from build123d import *

# Parameters (mm, degrees)
SKETCH1_W           = 35
SKETCH1_H           = 46
BOSS_EXTRUDE1_DEPTH = 13
SKETCH2_R           = 1.65
CUT_EXTRUDE1_DEPTH  = 26
SKETCH5_R           = 10.2
CUT_EXTRUDE2_DEPTH  = 46
SKETCH8_R           = 1.65
CUT_EXTRUDE3_DEPTH  = 26
SKETCH9_R           = 1.65
CUT_EXTRUDE4_DEPTH  = 35


with BuildPart() as part:
    # Sketch1 → Boss-Extrude1 (new body, symmetric)
    with BuildSketch(Plane(origin=(0, 0, 0), x_dir=(1, 0, 0), z_dir=(0, 1, 0))):
        Rectangle(SKETCH1_W, SKETCH1_H)
    extrude(amount=BOSS_EXTRUDE1_DEPTH, both=True)

    # Sketch2 → Cut-Extrude1 (cut)
    with BuildSketch(Plane(origin=(0, 13, 0), x_dir=(1, 0, 0), z_dir=(0, 1, 0))):
        with Locations((-13.5, 3)):
            Circle(SKETCH2_R)
        with Locations((-13.5, -19)):
            Circle(SKETCH2_R)
        with Locations((13.5, -19)):
            Circle(SKETCH2_R)
        with Locations((13.5, 3)):
            Circle(SKETCH2_R)
    extrude(amount=-CUT_EXTRUDE1_DEPTH, mode=Mode.SUBTRACT)

    # Sketch5 → Cut-Extrude2 (cut)
    with BuildSketch(Plane.XY.offset(23)):
        Circle(SKETCH5_R)
    extrude(amount=-CUT_EXTRUDE2_DEPTH, mode=Mode.SUBTRACT)

    # Sketch8 → Cut-Extrude3 (cut)
    with BuildSketch(Plane(origin=(0, 13, 0), x_dir=(1, 0, 0), z_dir=(0, 1, 0))):
        with Locations((0, 15)):
            Circle(SKETCH8_R)
    extrude(amount=-CUT_EXTRUDE3_DEPTH, mode=Mode.SUBTRACT)

    # Sketch9 → Cut-Extrude4 (cut)
    with BuildSketch(Plane.ZY.offset(17.5)):
        with Locations((7, 0)):
            Circle(SKETCH9_R)
    extrude(amount=-CUT_EXTRUDE4_DEPTH, mode=Mode.SUBTRACT)


solid = part.part
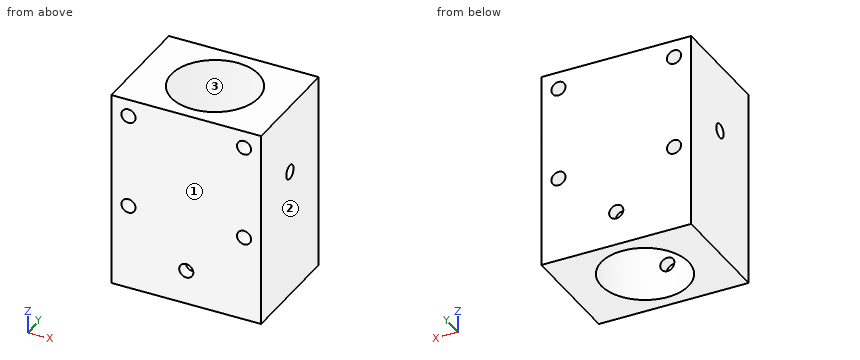
Work out the finished part from the listing and answer in its coordinate system (mm). Face numbers are marked on the shaded views. Round coordinates to 2 decimals unless told otherwise and drop trailing zeros. Loops run counter-clockwise (first coordinate to the right, second up) from the corner with the lowest first, then second, coordinate; pieces in that order, holes last. Notation, with made-up numbers: (71, 76) - (117, 76) arc R13 ccw to (117, 99) - close; hole circle Ø3 at (13, -0.75). An arc over 180 degrees is marked (long way). Use one line per item in the form item = value. Start each with the question number.
(1) Find section D-D on x = 0. Determine the outline of the cut face in (y, z), and give its area (3 significant figures).
(2) Find section B-B on x = -13.5. Determine the outline of the cut face in (y, z).
(3) Consider line 1 (Y direction, x = 0, z = -11); line 2 (Z direction, x = -13.5, y = -5); line 3 (Y direction, x = -1.5, z = 10). Determine where each line is inside the solid, lowest interval first.
(4) Determine the mould class of the marked faces 1, 2 and 3 for opening direction X: +X half, -X half, draft (parallel to the pull), parting line (faces both ways), or undercut.
(5) A flat-ended cylindrical pin translates along its axis: P1, Ø3, axis at y = 0, z = 7, coming from the +X side. Find the tip coordinate at first contact, or state that the pin passes through.
(6) Find section A-A on y = 0. Determine the outline of the cut face in (x, z).
(7) Find section C-C on z = 19. Determine the outline of the cut face in (x, y).
Answer list:
q1.outline = (-13, -23) - (-10.2, -23) - (-10.2, -16.65) - (-13, -16.65) - close; (-13, -13.35) - (-10.2, -13.35) - (-10.2, 23) - (-13, 23) - close; (10.2, -23) - (13, -23) - (13, -16.65) - (10.2, -16.65) - close; (10.2, -13.35) - (13, -13.35) - (13, 23) - (10.2, 23) - close
q1.area = 239 mm^2
q2.outline = (-13, -23) - (13, -23) - (13, -4.65) - (-13, -4.65) - close; (-13, -1.35) - (13, -1.35) - (13, 17.35) - (-13, 17.35) - close; (-13, 20.65) - (13, 20.65) - (13, 23) - (-13, 23) - close; hole circle Ø3.3 at (0, 7)
q3.line_1 = -13 to -10.2, 10.2 to 13
q3.line_2 = -23 to -4.65, -1.35 to 17.35, 20.65 to 23
q3.line_3 = -13 to -10.09, 10.09 to 13
q4.face_1 = draft
q4.face_2 = +X half
q4.face_3 = undercut
q5.P1 = through
q6.outline = (-17.5, -23) - (-10.2, -23) - (-10.2, 5.35) - (-17.5, 5.35) - close; (-17.5, 8.65) - (-10.2, 8.65) - (-10.2, 23) - (-17.5, 23) - close; (10.2, -23) - (17.5, -23) - (17.5, 5.35) - (10.2, 5.35) - close; (10.2, 8.65) - (17.5, 8.65) - (17.5, 23) - (10.2, 23) - close; hole circle Ø3.3 at (-13.5, -3); hole circle Ø3.3 at (-13.5, 19); hole circle Ø3.3 at (13.5, -3); hole circle Ø3.3 at (13.5, 19)
q7.outline = (-17.5, -13) - (-15.15, -13) - (-15.15, 13) - (-17.5, 13) - close; (-11.85, -13) - (11.85, -13) - (11.85, 13) - (-11.85, 13) - close; (15.15, -13) - (17.5, -13) - (17.5, 13) - (15.15, 13) - close; hole circle Ø20.4 at (0, 0)
